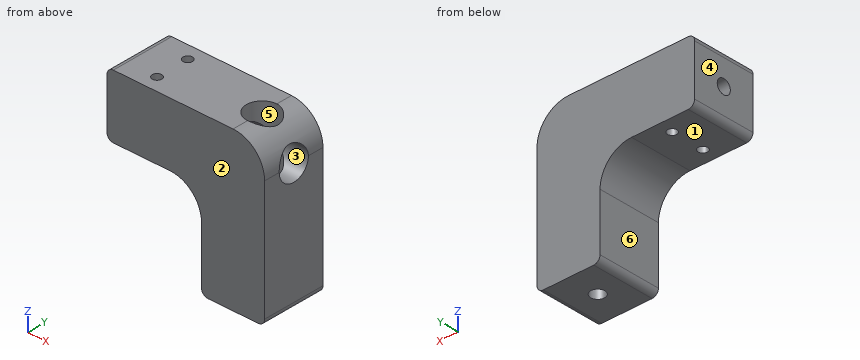
```python
from build123d import *

# Parameters (mm, degrees)
BOSS_EXTRUDE1_DEPTH = 10
SKETCH2_R           = 2.25
CUT_EXTRUDE1_DEPTH  = 65.807406984
SKETCH3_R           = 2.25
CUT_EXTRUDE2_DEPTH  = 60.160797831
SKETCH5_R           = 5
CUT_EXTRUDE3_DEPTH  = 42
SKETCH6_R           = 5
CUT_EXTRUDE4_DEPTH  = 42
CHAMFER1_SIZE       = 2.75
FILLET1_R           = 10
FILLET2_R           = 2
SKETCH8_R           = 1.5
CUT_EXTRUDE5_DEPTH  = 28


# Some blends are built 0.0001 mm under size
with BuildPart() as part:
    # Sketch1 → Boss-Extrude1 (new, symmetric)
    with BuildSketch(Plane(origin=(0, 0, 0), x_dir=(1, 0, 0), z_dir=(0, 1, 0))):
        Polygon((-10, 30), (10, 30), (10, -20), (-40, -20), (-40, 0), (-10, 0), align=None)
    extrude(amount=BOSS_EXTRUDE1_DEPTH, both=True)

    # Sketch2 → Cut-Extrude1 (cut, through all)
    with BuildSketch(Plane(origin=(0, 0, -30), x_dir=(-1, 0, 0), z_dir=(0, 0, -1))):
        Circle(SKETCH2_R)
    extrude(amount=-CUT_EXTRUDE1_DEPTH, mode=Mode.SUBTRACT)

    # Sketch3 → Cut-Extrude2 (cut, through all)
    with BuildSketch(Plane.ZY.offset(40)):
        with Locations((10, 0)):
            Circle(SKETCH3_R)
    extrude(amount=-CUT_EXTRUDE2_DEPTH, mode=Mode.SUBTRACT)

    # Sketch5 → Cut-Extrude3 (cut)
    with BuildSketch(Plane.XY.offset(20)):
        Circle(SKETCH5_R)
    extrude(amount=-CUT_EXTRUDE3_DEPTH, mode=Mode.SUBTRACT)

    # Sketch6 → Cut-Extrude4 (cut)
    with BuildSketch(Plane.ZY.offset(-10)):
        with Locations(Location((10, 0, 0), (0, 0, 180))):
            Circle(SKETCH6_R)
    extrude(amount=CUT_EXTRUDE4_DEPTH, mode=Mode.SUBTRACT)

    # Chamfer1
    chamfer1_edges = [part.edges().sort_by_distance(p)[0] for p in [
        (2.25, 0, -22),
        (-32, 0, 7.75),
    ]]
    chamfer(chamfer1_edges, length=CHAMFER1_SIZE - 0.0001)  # a hair under: the kernel refuses the full size

    # Fillet1
    # the kernel refuses this fillet: 10 mm, written as the material it adds along each edge
    with BuildSketch(Plane(origin=(-10, -10, 0), x_dir=(0, 0, -1), z_dir=(0, 1, 0))) as fillet1_piece_1:
        with BuildLine():
            CenterArc((FILLET1_R, FILLET1_R), FILLET1_R, 180, 90)
            Line((0, FILLET1_R), (0, 0))
            Line((0, 0), (FILLET1_R, 0))
        make_face()
    extrude(amount=20)
    # the kernel refuses this fillet: 10 mm, written as the material it takes off along each edge
    with BuildSketch(Plane(origin=(10, 35, 20), x_dir=(0, 0, -1), z_dir=(0, -1, 0))) as fillet1_2_piece_1:
        with BuildLine():
            CenterArc((FILLET1_R, -FILLET1_R), FILLET1_R, 90, 90)
            Line((0, -FILLET1_R), (0, 0))
            Line((0, 0), (FILLET1_R, 0))
        make_face()
    extrude(amount=70, mode=Mode.SUBTRACT)

    # Fillet2
    fillet2_edges = [part.edges().sort_by_distance(p)[0] for p in [
        (-10, 0, -30),
        (10, 0, -30),
        (-40, 0, 20),
        (-40, 0, 0),
    ]]
    fillet(fillet2_edges, radius=FILLET2_R)

    # Sketch8 → Cut-Extrude5 (cut)
    with BuildSketch(Plane.XY.offset(20)):
        with Locations((-28.509155223, 5.263420724)):
            Circle(SKETCH8_R)
        with Locations((-28.509155223, -5.263420724)):
            Circle(SKETCH8_R)
    extrude(amount=-CUT_EXTRUDE5_DEPTH, mode=Mode.SUBTRACT)


solid = part.part
```
The model under review builds one solid part; all positions refer to its coordinate system, in mm. Face numbers are marked on the shaded views. A direction names the side the tool comes from. Round coordinates to 2 decimals unless told otherwise and drop trailing zeros. Loops run counter-clockwise (first coordinate to the right, second up) from the corner with the lowest first, then second, coordinate; pieces in that order, holes last. Notation, with made-up numbers: (84, 71) -> (102, 71) arc R24 cw to (102, 96) -> close; hole circle Ø6 at (55.25, 36.5). An arc over 180 degrees is marked (long way). Answer in a Markdown table with one row per item.
1) Consider section A-A, the plane z = -18.5. Write out the cut boundary in (x, y), plus the area to 3 significant figures.
Taken from the geometry:
| item | result |
|---|---|
| outline | (-10, -10) -> (10, -10) -> (10, 10) -> (-10, 10) -> close; hole circle Ø10 at (0, 0) |
| area | 321 mm² |
2) Consider section B-B, the plane y = -7.5. Write out the cut boundary in (x, z), plus the area to 3 significant figures.
Taken from the geometry:
| item | result |
|---|---|
| outline | (-40, 2) arc R2 ccw to (-38, 0) -> (-20, 0) arc R10 cw to (-10, -10) -> (-10, -28) arc R2 ccw to (-8, -30) -> (8, -30) arc R2 ccw to (10, -28) -> (10, 10) arc R10 ccw to (0, 20) -> (-38, 20) arc R2 ccw to (-40, 18) -> close |
| area | 1,600 mm² |
3) Consider section C-C, the plane y = 0. Count the separate pieces of the cut face and the enclosed holes in it, plus the area to 3 significant figures.
Taken from the geometry:
| item | result |
|---|---|
| separate pieces | 4 |
| enclosed holes | 0 |
| area | 774 mm² |
4) For pin 1 Ø6 at (x, y) = (0, 0) entering from -Z; pin 2 Ø2.5 at (x, y) = (-28.51, 5.26) entering from +Z; pin 3 Ø5.5 at (y, z) = (-0.5, -16.5) entering from -X; pin 4 Ø3 at (x, y) = (1.5, -2.5) entering from +Z, all flat-tipped, find the tip position at first contact; note any pin that passes through.
Taken from the geometry:
| item | result |
|---|---|
| pin 1 | stops at z = -30 |
| pin 2 | passes through |
| pin 3 | stops at x = -10 |
| pin 4 | stops at z = -22.58 |
5) Draft analysis for pull direction Z (two halves, no side actions). For the marked faces 1, 2 and 3, state which applies: pulls with the +Z half, pulls with the -Z half, needs draft (parallel to the pull), parting line crosses it, or undercut.
Taken from the geometry:
| item | result |
|---|---|
| face 1 | pulls with the -Z half |
| face 2 | needs draft |
| face 3 | undercut |
6) Wall thickness on line 1 along X through (y, z) = (0, 16); line 2 along X through (y, z) = (-4.5, 3); line 3 along Z through (x, y) = (-24, -6.75): over which ranges is each line inside the solid? List them lowest first.
Taken from the geometry:
| item | result |
|---|---|
| line 1 | x = -40 to -5, 5 to 8 |
| line 2 | x = -40 to -29.8, -27.22 to -2.18, 2.18 to 10 |
| line 3 | z = 0 to 20 |
7) Tool access review of the marked faces 4, 5 and 6: name each direction out of +Z, -Z, +X, -X, +Y, -Y from which nothing blocks a thin tool from reaching the whole face with its end or side.
Taken from the geometry:
| item | result |
|---|---|
| face 4 | +Z, -Z, -X, +Y, -Y |
| face 5 | +Z |
| face 6 | -Z, -X, +Y, -Y |
8) Consider section D-D, the plane x = 6.5. Write out the cut boundary in (y, z), plus the area to 3 significant figures.
Taken from the geometry:
| item | result |
|---|---|
| outline | (-10, -30) -> (10, -30) -> (10, 17.6) -> (-10, 17.6) -> close; hole circle Ø10 at (0, 10) |
| area | 873 mm² |
